Check sheet for the drawn part. Datum: minimum x, y, z corner. Units: mm. A direction names the side the tool comes from. Coordinates: 2 decimals unless noted, no trailing zeros. Order: outer loops, then holes, each group sorted by start corner. A loop starts at its lowest first (then second) coordinate and runs counter-clockwise, first axis right, second up. Notation, with made-up numbers: (42, 22) - (93, 22) arc R30 ccw to (93, 59) - close; hole circle Ø8 at (86, 66.25). An arc over 180 degrees is marked (long way). Put each result on its own line as item: value.
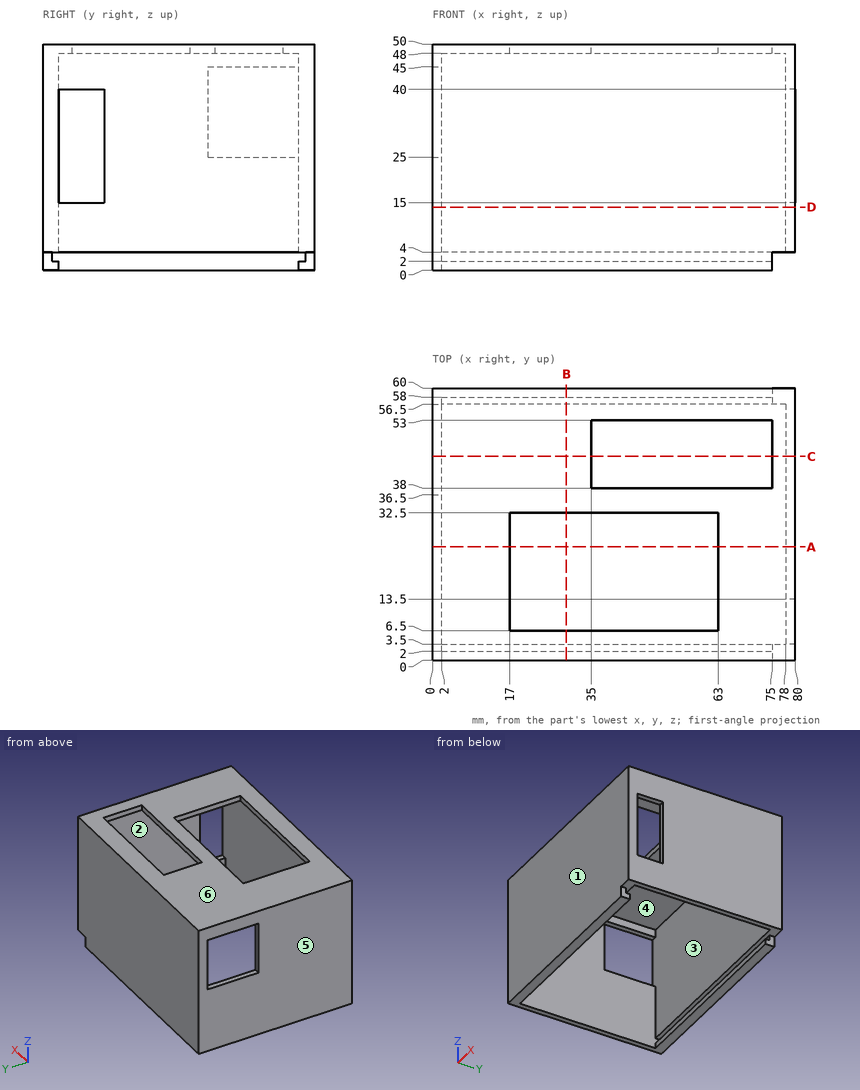
Q1. Section check C-C on y = 45. Record the boundary of the cut face in (x, z).
Answer block:
outline: (0, 0) - (2, 0) - (2, 25) - (0, 25) - close; (0, 45) - (2, 45) - (2, 48) - (35, 48) - (35, 50) - (0, 50) - close; (75, 48) - (78, 48) - (78, 4) - (80, 4) - (80, 50) - (75, 50) - close
Q2. Thickness scan on L1, parallel to Y at x = 4, z = 22; L2, parallel to Z at x = 17, y = 57; L3, parallel to X at y = 13.5, z = 40.5. Record the ranges inside material, lowest first. Write a range as [from, to].
Answer block:
L1: y = [0, 3.5], [56.5, 60]
L2: z = [0, 2], [4, 50]
L3: x = [0, 2], [78, 80]
Q3. Draft check along X on the marked faces 3, 4, 5 and 6. Enter one of: pulls with the +X half, pulls with the -X half, needs draft (parallel to the pull), parting line crosses it, or undercut.
Answer block:
face 3: undercut
face 4: undercut
face 5: pulls with the -X half
face 6: needs draft
Q4. Section check B-B on x = 29.5. Record the boundary of the cut face in (y, z), then the cut area to 3 significant figures.
Answer block:
outline: (0, 0) - (3.5, 0) - (3.5, 2) - (2, 2) - (2, 4) - (3.5, 4) - (3.5, 48) - (6.5, 48) - (6.5, 50) - (0, 50) - close; (32.5, 48) - (56.5, 48) - (56.5, 4) - (58, 4) - (58, 2) - (56.5, 2) - (56.5, 0) - (60, 0) - (60, 50) - (32.5, 50) - close
area: 398 mm^2
Q5. Access from +Z, -Z, +X, -X, +Y, -Y to the whole of each face (thin tool, end or side, straight path). Record for the marked faces 1 and 2.
Answer block:
face 1: +Z, -Z, +X, -X, -Y
face 2: -Z
Q6. Section check A-A on y = 25. Record the boundary of the cut face in (x, z).
Answer block:
outline: (0, 0) - (2, 0) - (2, 48) - (17, 48) - (17, 50) - (0, 50) - close; (63, 48) - (78, 48) - (78, 4) - (80, 4) - (80, 50) - (63, 50) - close
Q7. Section check D-D on z = 14. Record the boundary of the cut face in (x, y).
Answer block:
outline: (0, 0) - (80, 0) - (80, 60) - (0, 60) - close; hole (2, 3.5) - (78, 3.5) - (78, 56.5) - (2, 56.5) - close
Q8. Depth check by flat-ended pin: pin 1 Ø1 at (x, y) = (71, 24.5) entering from -Z; pin 2 Ø1 at (y, z) = (58, 1.5) entering from +X; pin 3 Ø4 at (y, z) = (41, 30.5) entering from -X. Enter the tip coordinate at first touch or a pass-through.
Answer block:
pin 1: stops at z = 48
pin 2: stops at x = 75
pin 3: stops at x = 78
